The model under review builds one solid part; all positions refer to its coordinate system, in mm. Coordinates: 2 decimals unless noted, no trailing zeros. Write each loop counter-clockwise with the first axis right and the second up, starting at its lowest first coordinate (ties: lowest second). Pieces come first, ordered by that corner, then holes. Notation, with made-up numbers: M -32,75 L -24,75 A28 cw -24,100 Z; hole C 80,-6 d10. An arc over 180 degrees is marked long. Answer as a JSON object with one key per item and string values.
```python
from build123d import *

# Parameters (mm, degrees)
SKETCH3_R           = 1.5
BOSS_EXTRUDE1_DEPTH = 1.35
FILLET1_R           = 2
FILLET2_R           = 3
FILLET3_R           = 5
SKETCH4_R           = 1.75
CUT_EXTRUDE1_DEPTH  = 86.197993521


with BuildPart() as part:
    # Sketch3 → Boss-Extrude1 (new body)
    with BuildSketch(Plane(origin=(0, 0, 0), x_dir=(1, 0, 0), z_dir=(0, 1, 0))):
        Polygon((31.305, 15.75), (31.305, 57.34), (-31.305, 57.34), (-31.305, 15.75), (-63, 15.75), (-63, -15.75), (-31.305, -15.75), (-31.305, -57.34), (31.305, -57.34), (31.305, -15.75), (63, -15.75), (63, 15.75), align=None)
        with Locations(Location((-57, 11.65, 0), (0, 0, 90))):
            Circle(SKETCH3_R, mode=Mode.SUBTRACT)
        with Locations(Location((-57, -11.65, 0), (0, 0, 90))):
            Circle(SKETCH3_R, mode=Mode.SUBTRACT)
        with Locations(Location((-37, -8.15, 0), (0, 0, 90))):
            Circle(SKETCH3_R, mode=Mode.SUBTRACT)
        with Locations(Location((-37, 8.15, 0), (0, 0, 90))):
            Circle(SKETCH3_R, mode=Mode.SUBTRACT)
        with Locations(Location((37, 8.15, 0), (0, 0, 90))):
            Circle(SKETCH3_R, mode=Mode.SUBTRACT)
        with Locations(Location((57, 11.65, 0), (0, 0, 90))):
            Circle(SKETCH3_R, mode=Mode.SUBTRACT)
        with Locations(Location((57, -11.65, 0), (0, 0, 90))):
            Circle(SKETCH3_R, mode=Mode.SUBTRACT)
        with Locations(Location((37, -8.15, 0), (0, 0, 90))):
            Circle(SKETCH3_R, mode=Mode.SUBTRACT)
        with Locations(Location((-13.5, 39.735100189, 0), (0, 0, 90))):
            Circle(SKETCH3_R, mode=Mode.SUBTRACT)
        with Locations(Location((13.5, 39.735100189, 0), (0, 0, 90))):
            Circle(SKETCH3_R, mode=Mode.SUBTRACT)
        with Locations(Location((-24.05, -50.064899811, 0), (0, 0, 90))):
            Circle(SKETCH3_R, mode=Mode.SUBTRACT)
        with Locations(Location((24.05, -50.064899811, 0), (0, 0, 90))):
            Circle(SKETCH3_R, mode=Mode.SUBTRACT)
    extrude(amount=BOSS_EXTRUDE1_DEPTH)

    # Fillet1
    fillet1_edges = [part.edges().sort_by_distance(p)[0] for p in [
        (63, 0.675, -15.75),
        (63, 0.675, 15.75),
        (-63, 0.675, 15.75),
        (-63, 0.675, -15.75),
    ]]
    fillet(fillet1_edges, radius=FILLET1_R)

    # Fillet2
    fillet2_edges = [part.edges().sort_by_distance(p)[0] for p in [
        (-31.305, 0.675, -57.34),
        (31.305, 0.675, -57.34),
        (31.305, 0.675, 57.34),
        (-31.305, 0.675, 57.34),
    ]]
    fillet(fillet2_edges, radius=FILLET2_R)

    # Fillet3
    fillet3_edges = [part.edges().sort_by_distance(p)[0] for p in [
        (-31.305, 0.675, -15.75),
        (31.305, 0.675, -15.75),
        (31.305, 0.675, 15.75),
        (-31.305, 0.675, 15.75),
    ]]
    fillet(fillet3_edges, radius=FILLET3_R)

    # Sketch4 → Cut-Extrude1 (cut, through all)
    with BuildSketch(Plane(origin=(0, 1.35, 0), x_dir=(1, 0, 0), z_dir=(0, 1, 0))):
        with Locations(Location((-21, -10.75, 0), (0, 0, 270))):
            Circle(SKETCH4_R)
        with Locations(Location((21, -10.75, 0), (0, 0, 270))):
            Circle(SKETCH4_R)
        with Locations(Location((21, 10.75, 0), (0, 0, 270))):
            Circle(SKETCH4_R)
        with Locations(Location((-21, 10.75, 0), (0, 0, 270))):
            Circle(SKETCH4_R)
    extrude(amount=-CUT_EXTRUDE1_DEPTH, mode=Mode.SUBTRACT)


solid = part.part
```
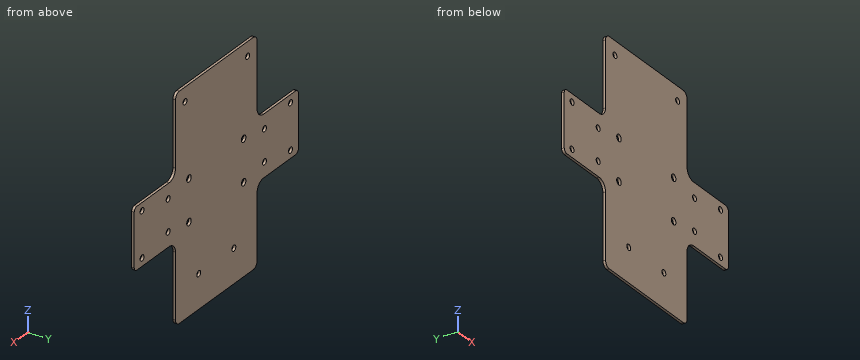
(1) Wall thickness on line 1 along Z through (x, y) = (-37, 0.3); line 2 along X through (y, z) = (1, 8.15); line 3 along Z through (x, y) = (13.5, 0.7): over which ranges is each line inside the solid? List them lowest first. Write a range as from..to.
Results list:
{"line 1": "-15.75..-9.65, -6.65..6.65, 9.65..15.75", "line 2": "-63..-38.5, -35.5..35.5, 38.5..63", "line 3": "-57.34..-41.24, -38.24..57.34"}
(2) Add section C-C on z = -29. Give the boundary of the cut face in (x, y) (3 decimals).
Results list:
{"outline": "M -31.305,0 L 31.305,0 L 31.305,1.35 L -31.305,1.35 Z"}
(3) For pin 1 Ø2.5 at (x, z) = (-24.05, 50.06) entering from +Y; pin 2 Ø0.7 at (y, z) = (0.5, -35.5) entering from -X (3 decimals); pin 3 Ø0.7 at (x, y) = (43, 0.5) entering from +Z, all flat-tipped, find the tip position at first contact; note any pin that passes through.
Results list:
{"pin 1": "through", "pin 2": "x = -31.305", "pin 3": "z = 15.75"}
(4) Add section B-B on x = -13.5. Give the boundary of the cut face in (y, z).
Results list:
{"outline": "M 0,-57.34 L 1.35,-57.34 L 1.35,-41.24 L 0,-41.24 Z; M 0,-38.24 L 1.35,-38.24 L 1.35,57.34 L 0,57.34 Z"}
(5) Add section D-D on y = 0.8. Count the separate pieces of the cut face and the enclosed holes in it, and give its area (3 significant figures).
Results list:
{"separate pieces": "1", "enclosed holes": "16", "area": "9,060 mm²"}
(6) Add section A-A on x = 57. Give the boundary of the cut face in (y, z).
Results list:
{"outline": "M 0,-15.75 L 1.35,-15.75 L 1.35,-13.15 L 0,-13.15 Z; M 0,-10.15 L 1.35,-10.15 L 1.35,10.15 L 0,10.15 Z; M 0,13.15 L 1.35,13.15 L 1.35,15.75 L 0,15.75 Z"}
